Source: CAD feature listing. Evaluate the final solid. Frame: model axes, mm. A direction names the side the tool comes from. Coordinates: 2 decimals unless noted, no trailing zeros. Order: outer loops, then holes, each group sorted by start corner. A loop starts at its lowest first (then second) coordinate and runs counter-clockwise, first axis right, second up.
```python
from build123d import *

# Parameters (mm, degrees)
CROQUIS1_R              = 59
SALIENTE_EXTRUIR1_DEPTH = 1.5
SALIENTE_EXTRUIR2_DEPTH = 1.5
ESCALA1_SCALE           = 0.8
CORTAR_EXTRUIR1_DEPTH   = 0.7


with BuildPart() as part:
    # Croquis1 → Saliente-Extruir1 (new body)
    with BuildSketch(Plane.XY):
        Circle(CROQUIS1_R)
    extrude(amount=SALIENTE_EXTRUIR1_DEPTH)

    # Croquis2 → Saliente-Extruir2 (add)
    with BuildSketch(Plane.XY.offset(1.5)):
        with BuildLine():
            Line((-62.713634881, 6), (62.713634881, 6))
            ThreePointArc((62.713634881, 6), (63, 0), (62.713634881, -6))
            Line((62.713634881, -6), (-62.713634881, -6))
            ThreePointArc((-62.713634881, -6), (-63, 0), (-62.713634881, 6))
        make_face()
    extrude(amount=-SALIENTE_EXTRUIR2_DEPTH)


with BuildPart() as part_1:
    # Escala1: scaled about (0, 0, 0.75)
    add(part.part.scale(ESCALA1_SCALE).moved(Location((0, 0, 0.15))))

    # Croquis7 → Cortar-Extruir1 (cut)
    with BuildSketch(Plane.XY.offset(1.35)):
        Polygon((-0.779467376, 0), (-0.779467376, 5.314550288), (-0.779467376, 18.352913661), (4.322500901, 18.352913661), (4.322500901, 5.314550288), (11.408567952, 5.314550288), (11.408567952, 0), align=None)
        Polygon((-15.801929523, 18.352913661), (-23.029717915, 0), (-16.79397891, 0), (-15.801929523, 2.657275144), (-9.566190518, 2.657275144), (-8.684228244, 0), (-2.338402127, 0), (-8.429821566, 18.352913661), align=None)
        Polygon((-10.617093295, 7.257317405), (-14.282649957, 7.257317405), (-12.115875544, 13.817830749), align=None, mode=Mode.SUBTRACT)
        Polygon((-24.872095348, 0), (-24.872095348, 13.817830749), (-19.770127071, 13.817830749), (-19.770127071, 18.352913661), (-35.359474583, 18.352913661), (-35.359474583, 13.817830749), (-30.257506306, 13.817830749), (-30.257506306, 0), align=None)
        Polygon((-24.872095348, -18.919799025), (-24.872095348, -5.925877823), (-19.770127071, -5.925877823), (-19.770127071, -0.941442838), (-35.359474583, -0.941442838), (-35.359474583, -5.925877823), (-30.257506306, -5.925877823), (-30.257506306, -18.919799025), align=None)
        Polygon((-4.281500949, -14.454799909), (-4.281500949, -18.919799025), (-18.34868413, -18.919799025), (-18.34868413, -0.941442838), (-4.281500949, -0.941442838), (-4.281500949, -5.925877823), (-12.115875544, -5.925877823), (-12.115875544, -7.587356151), (-4.281500949, -7.587356151), (-4.281500949, -12.461025915), (-12.115875544, -12.461025915), (-12.115875544, -14.454799909), align=None)
        with BuildLine():
            ThreePointArc((10.477188742, -8.24524686), (2.187062141, -10.245721477), (10.477188742, -12.246196094))
            Line((10.477188742, -12.246196094), (15.133105793, -14.632150132))
            ThreePointArc((15.133105793, -14.632150132), (-3.044604921, -10.245721477), (15.133105793, -5.859292822))
            Line((15.133105793, -5.859292822), (10.477188742, -8.24524686))
        make_face()
        Polygon((28.394239509, -12.461025915), (28.394239509, -18.919799025), (33.800539832, -18.919799025), (33.800539832, -0.941442838), (28.394239509, -0.941442838), (28.394239509, -6.756616987), (21.748326196, -6.756616987), (21.748326196, -0.941442838), (16.210065101, -0.941442838), (16.210065101, -18.919799025), (21.748326196, -18.919799025), (21.748326196, -12.461025915), align=None)
    extrude(amount=-CORTAR_EXTRUIR1_DEPTH, mode=Mode.SUBTRACT)


solid = part_1.part
```
1. Section query A-A on z = 0.45. Return loops of the section in (x, y), plus the area to 3 significant figures.
Findings:
outline: (-50.17, -4.8) - (-46.96, -4.8) arc R47.2 ccw to (46.96, -4.8) - (50.17, -4.8) arc R50.4 ccw to (50.17, 4.8) - (46.96, 4.8) arc R47.2 ccw to (-46.96, 4.8) - (-50.17, 4.8) arc R50.4 ccw to start
area: 7,060 mm2
2. Section query C-C on y = 32.5. Return loops of the section in (x, z), plus the area to 3 significant figures.
Findings:
outline: (-34.23, 0.15) - (34.23, 0.15) - (34.23, 1.35) - (-34.23, 1.35) - close
area: 82.1 mm2
3. Pin query (flat end, axial travel): P1, Ø0.6, axis at x = -9, z = 1, coming from the -Y side; P2, Ø0.6, axis at y = 13.5, z = 1, coming from the -X side. Return the tip coordinate at first contact, or that it passes through.
Findings:
P1: stops at y = -46.39
P2: stops at x = -45.32
4. Section query D-D on x = 9. Return loops of the section in (y, z).
Findings:
outline: (-46.33, 0.15) - (46.33, 0.15) - (46.33, 1.35) - (5.31, 1.35) - (5.31, 0.65) - (0, 0.65) - (0, 1.35) - (-0.94, 1.35) - (-0.94, 0.65) - (-6.59, 0.65) - (-6.59, 1.35) - (-13.9, 1.35) - (-13.9, 0.65) - (-19.55, 0.65) - (-19.55, 1.35) - (-46.33, 1.35) - close
5. Access query for faces 1 (the face through (1, 1, 0.15)), 2 (the face through (-5.341, 9.048, 1.005)). Directions: +Z, -Z, +X, -X, +Y, -Y. A direction counts if a zero-diameter tool reaches every point of the face in a straight line with its end or side. Return the directions, or none.
Findings:
face 1: -Z, +X, -X, +Y, -Y
face 2: +Z
6. Draft query along Y for faces 3 (the face through (-0.97, -47.19, 0.74)), 4 (the face through (-12, 9, 1.35)), 5 (the face through (-11, -10, 0.65)), 6 (the face through (2, -10, 0.65)). Return one class per face: released by +Y, released by -Y, zero draft, split by the parting line, or undercut.
Findings:
face 3: released by -Y
face 4: zero draft
face 5: undercut
face 6: undercut
7. Section query B-B on x = 25.5. Return loops of the section in (y, z), plus the area to 3 significant figures.
Findings:
outline: (-39.72, 0.15) - (39.72, 0.15) - (39.72, 1.35) - (-6.76, 1.35) - (-6.76, 0.65) - (-12.46, 0.65) - (-12.46, 1.35) - (-39.72, 1.35) - close
area: 91.3 mm2
8. Ray query, line 1 (X direction, y = -16, z = 0.8); line 2 (X direction, y = 17, z = 1.15); line 3 (Y direction, x = 4, z = 0.9). Return the intervals inside material, ascending.
Findings:
line 1: x = -44.41 to -30.26, -24.87 to -18.35, -4.28 to -1.13, 14.28 to 16.21, 21.75 to 28.39, 33.8 to 44.41
line 2: x = -44.03 to -35.36, -19.77 to -16.33, -7.98 to -0.78, 4.32 to 44.03
line 3: y = -47.03 to -19.51, -13.8 to -6.69, -0.98 to 0, 18.35 to 47.03
